Geometry: final body of the model. Coordinates: model frame, mm. Face numbers are marked on the shaded views. Coordinates: 2 decimals unless noted, no trailing zeros. Order: outer loops, then holes, each group sorted by start corner. A loop starts at its lowest first (then second) coordinate and runs counter-clockwise, first axis right, second up. Notation, with made-up numbers: M 15,14.5 L 41,14.5 A24 ccw 41,49.5 Z; hole C -15.5,30 d10. An arc over 180 degrees is marked long. Use CSV: the item, a comma, the result in double quotes. Start each with the question number.
Q1. Mould query, pull axis Z, two halves, no side actions, for the marked faces 1, 2 and 3. Classes: +Z half, -Z half, draft (parallel to the pull), parting line (faces both ways), or undercut.
Q2. Section query C-C, the plane y = 23.5. Output: boundary loops of the cut face in (x, z), and give its area (3 significant figures).
Q3. Section query D-D, the plane x = -16.5. Output: boundary loops of the cut face in (y, z).
Q4. Ray query, probe 1 along X at (y, z) = (7.5, 0); probe 2 along Y at (x, z) = (-11, 13); probe 3 along Z at (x, y) = (-1, 6.5). Return the intervals inside material, ascending.
Q5. First-contact query: P1, Ø3, axis at x = -4.5, y = 23.5, coming from the +Z side; P2, Ø6, axis at x = -8, y = 8.5, coming from the +Z side; P3, Ø12, axis at y = 4, z = -8, coming from the +X side. Flat tips, straight axial feed; report the tip coordinate or a pass-through.
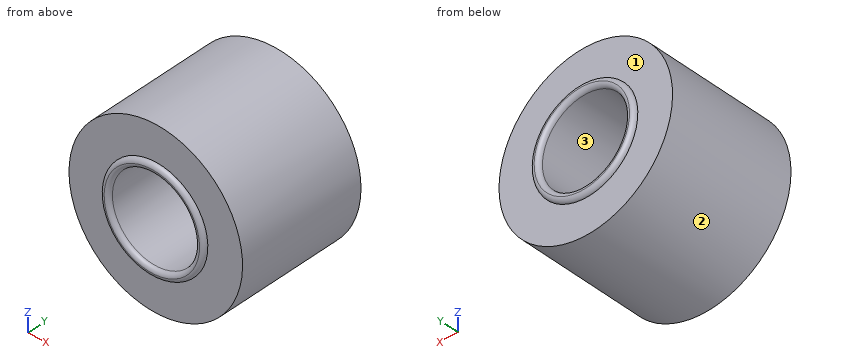
from build123d import *

# Parameters (mm, degrees)
PROFILE_SKETCH_R              = 20
PROFILE_SKETCH_R_2            = 10
PROFILE_EXTRUDE_DEPTH         = 30
RING_LIP_PROFILE_R            = 12
RING_LIP_PROFILE_R_2          = 10
TOP_RING_LIP_EXTRUDE_DEPTH    = 1
BOTTOM_START                  = -31
SKETCH2_2_R                   = 12
SKETCH2_2_R_2                 = 10
BOTTOM_RING_LIP_EXTRUDE_DEPTH = 1
TOP_RING_LIP_FILLET_R         = 1
BOTTOM_RING_LIP_FILLET_R      = 1


with BuildPart() as part:
    # Profile Sketch → Profile Extrude (new body)
    with BuildSketch(Plane(origin=(0, 0, 0), x_dir=(1, 0, 0), z_dir=(0, 1, 0))):
        with Locations(Location((0, 0, 0), (0, 0, 270))):
            Circle(PROFILE_SKETCH_R)
        with Locations(Location((0, 0, 0), (0, 0, 270))):
            Circle(PROFILE_SKETCH_R_2, mode=Mode.SUBTRACT)
    extrude(amount=PROFILE_EXTRUDE_DEPTH)

    # Ring Lip Profile → Top Ring Lip Extrude (add)
    with BuildSketch(Plane(origin=(0, 30, 0), x_dir=(1, 0, 0), z_dir=(0, 1, 0))):
        with Locations(Location((0, 0, 0), (0, 0, 270))):
            Circle(RING_LIP_PROFILE_R)
        with Locations(Location((0, 0, 0), (0, 0, 270))):
            Circle(RING_LIP_PROFILE_R_2, mode=Mode.SUBTRACT)
    extrude(amount=TOP_RING_LIP_EXTRUDE_DEPTH)

    # Sketch2<2> → Bottom Ring Lip Extrude (add)
    with BuildSketch(Plane(origin=(0, 30, 0), x_dir=(1, 0, 0), z_dir=(0, 1, 0)).offset(BOTTOM_START)):
        with Locations(Location((0, 0, 0), (0, 0, 270))):
            Circle(SKETCH2_2_R)
        with Locations(Location((0, 0, 0), (0, 0, 270))):
            Circle(SKETCH2_2_R_2, mode=Mode.SUBTRACT)
    extrude(amount=BOTTOM_RING_LIP_EXTRUDE_DEPTH)

    # Top Ring Lip Fillet
    top_ring_lip_fillet_edges = [part.edges().sort_by_distance(p)[0] for p in [
        (0, -1, -12),
        (0, -1, -10),
    ]]
    fillet(top_ring_lip_fillet_edges, radius=TOP_RING_LIP_FILLET_R - 0.0001)  # a hair under: the kernel refuses the full size

    # Bottom Ring Lip Fillet
    bottom_ring_lip_fillet_edges = [part.edges().sort_by_distance(p)[0] for p in [
        (0, 31, -12),
        (0, 31, -10),
    ]]
    fillet(bottom_ring_lip_fillet_edges, radius=BOTTOM_RING_LIP_FILLET_R - 0.0001)  # a hair under: the kernel refuses the full size


solid = part.part
Responses:
1,face 1,"draft"
1,face 2,"parting line"
1,face 3,"undercut"
2,outline,"C 0,0 d40; hole C 0,0 d20"
2,area,"942 mm²"
3,outline,"M 0,-11.3 L 30,-11.3 L 30,11.3 L 0,11.3 Z"
4,probe 1,"x = -20 to -10, 10 to 20"
4,probe 2,"y = 0 to 30"
4,probe 3,"z = -19.97 to -9.95, 9.95 to 19.97"
5,P1,"stops at z = 19.77"
5,P2,"stops at z = 19.36"
5,P3,"stops at x = 19.9"
